Autodesk Inventor part; units mm, degrees
ref_plane "YZ Plane" through (0, 0, 0) normal (1, 0, 0) x (0, 1, 0)
ref_plane "XZ Plane" through (0, 0, 0) normal (0, 1, 0) x (-1, 0, 0)
ref_plane "XY Plane" through (0, 0, 0) normal (0, 0, 1) x (1, 0, 0)
sketch "Sketch1" plane through (0, 0, 0) normal (0, 1, 0) x (-1, 0, 0)
  circle A0 centre (0, 0) radius 45
  dimension "d0" = 90
extrude "Extrusion1" add sketch "Sketch1" along normal blind 13
sketch "Sketch2" plane through (0, 0, 0) normal (0, 1, 0) x (-1, 0, 0)
  circle A0 centre (0, 0) radius 10
  line L0 (0, 0) -> (-40, 0)
  line L1 (0, 0) -> (-32.7661, -22.9431)
  arc A1 (-20, 0) -> (-16.383, -11.4715) centre (0, 0) ccw
  arc A2 (-40, 0) -> (-32.7661, -22.9431) centre (0, 0) ccw
  dimension "d3" = 20
  dimension "d5" = 35
  dimension "d16" = 40
extrude "Extrusion2" cut sketch "Sketch2" along normal blind 13 contours A0 L1 L0 | L0 L1 A0 | A1 L1 A2 L0
pattern_circular "Circular Pattern1" count 6 over 360 about axis through (0, 0, 0) along (0, 1, 0) of "Extrusion2"
properties part number "Brushless Motor Case"
Geometry: final body of the model. Coordinates: model frame, mm. Give positions to 0.01 mm unless a question says otherwise; leave off trailing zeros. Write each loop counter-clockwise with the first axis right and the second up, starting at its lowest first coordinate (ties: lowest second). Pieces come first, ordered by that corner, then holes. Notation, with made-up numbers: (37, 5.25) -> (81, 5.25) arc R22 cw to (81, 19.25) -> close; hole circle Ø6 at (-10, 33). An arc over 180 degrees is marked (long way). Answer as a JSON object with one key per item and string values.
1. Cut plane C-C on x = 13. Output: boundary loops of the cut face in (y, z).
Ans:
{"outline": "(0, -43.08) -> (13, -43.08) -> (13, -37.83) -> (0, -37.83) -> close; (0, -22.52) -> (13, -22.52) -> (13, 15.2) -> (0, 15.2) -> close; (0, 22.52) -> (13, 22.52) -> (13, 43.08) -> (0, 43.08) -> close"}
2. Ray query, probe 1 along Z at (x, y) = (-0.5, 6.75); probe 2 along X at (y, z) = (11.75, -3); probe 3 along X at (y, z) = (3, -17.5). Return the intervals inside material, ascending. Write a range as from..to.
Ans:
{"probe 1": "z = -45..-40, -19.99..-9.99, 9.99..19.99, 40..45", "probe 2": "x = -44.9..-9.54, 9.54..19.77, 39.89..44.9", "probe 3": "x = -41.46..-35.97, -10.1..9.68, 10.1..24.99, 35.97..41.46"}
3. Cut plane A-A on x = 0. Output: boundary loops of the cut face in (y, z), and give its area (3 significant figures).
Ans:
{"outline": "(0, -45) -> (13, -45) -> (13, -40) -> (0, -40) -> close; (0, -20) -> (13, -20) -> (13, -10) -> (0, -10) -> close; (0, 10) -> (13, 10) -> (13, 20) -> (0, 20) -> close; (0, 40) -> (13, 40) -> (13, 45) -> (0, 45) -> close", "area": "390 mm^2"}
4. Contact query for flat-ended pins moving along their axis: pin 1 (1.5 mm diameter, centred on x = 28.5, y = 11, fed in from +Z); pin 2 (3 mm diameter, centred on x = 23.5, y = 8.5, fed in from -Z); pin 3 (6 mm diameter, centred on y = 11, z = 20.5, fed in from -X); pin 4 (10 mm diameter, centred on x = -11.5, z = -22, fed in from -Y). Output: stop coordinate, or through.
Ans:
{"pin 1": "stops at z = 35.43", "pin 2": "stops at z = -39.26", "pin 3": "stops at x = -41.46", "pin 4": "stops at y = 0"}
5. Mould query, pull axis Z, two halves, no side actions, for faces 1 (the cylindrical face through (-19.048, 6.409, 6.096)), 2 (the flat face through (1, 0, 11)). Classes: pulls with the +Z half, pulls with the -Z half, needs draft (parallel to the pull), parting line crosses it, or undercut.
Ans:
{"face 1": "undercut", "face 2": "needs draft"}
6. Cut plane B-B on y = 5.25. Output: boundary loops of the cut face in (x, z), and give its area (3 significant figures).
Ans:
{"outline": "circle Ø90 at (0, 0); hole (-40, 0) -> (-20, 0) arc R20 cw to (-16.38, 11.47) -> (-32.77, 22.94) arc R40 ccw to start; hole (-36.25, -16.9) arc R40 ccw to (-20, -34.64) -> (-10, -17.32) arc R20 cw to (-18.13, -8.45) -> close; hole (-20, 34.64) -> (-10, 17.32) arc R20 cw to (1.74, 19.92) -> (3.49, 39.85) arc R40 ccw to start; hole circle Ø20 at (0, 0); hole (-3.49, -39.85) arc R40 ccw to (20, -34.64) -> (10, -17.32) arc R20 cw to (-1.74, -19.92) -> close; hole (10, 17.32) arc R20 cw to (18.13, 8.45) -> (36.25, 16.9) arc R40 ccw to (20, 34.64) -> close; hole (16.38, -11.47) -> (32.77, -22.94) arc R40 ccw to (40, 0) -> (20, 0) arc R20 cw to start", "area": "3,850 mm^2"}
